Here's how the part is built. I have some questions about the finished solid (model axes, mm). Face numbers are marked on the shaded views. A direction names the side the tool comes from. Give positions to 0.01 mm unless a question says otherwise; leave off trailing zeros. Write each loop counter-clockwise with the first axis right and the second up, starting at its lowest first coordinate (ties: lowest second). Pieces come first, ordered by that corner, then holes. Notation, with made-up numbers: (-31, 66.25) -> (10, 66.25) arc R25 ccw to (10, 97.25) -> close; hole circle Ø4 at (69.5, 8). An arc over 180 degrees is marked (long way). Return JSON: item names as keys, results as strings.
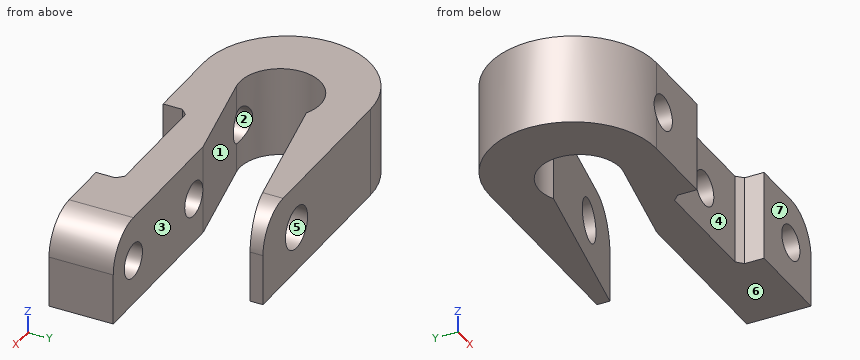
from build123d import *

# Parameters (mm, degrees)
BOSS_EXTRUDE1_DEPTH = 7
CUT_EXTRUDE1_REACH  = 28.495
SKETCH2_R           = 1.35
CUT_EXTRUDE2_REACH  = 28.495
SKETCH3_R           = 1.65
FILLET1_R           = 3
CHAMFER2_SIZE       = 0.5


with BuildPart() as part:
    # Sketch1 → Boss-Extrude1 (new body)
    with BuildSketch(Plane.XY):
        with BuildLine():
            Line((1.443086969, 2.8), (15, 5.5))
            Line((15, 5.5), (15, 6.5))
            Line((15, 6.5), (-1, 6.5))
            ThreePointArc((-1, 6.5), (-7.5, 0), (-1, -6.5))
            Line((-1, -6.5), (5, -6.5))
            Line((5, -6.5), (5, -4.5))
            Line((5, -4.5), (15, -4.5))
            Line((15, -4.5), (15, -6.5))
            Line((15, -6.5), (22, -6.5))
            Line((22, -6.5), (22, -1.5))
            Line((22, -1.5), (8.595407496, -1.5))
            Line((8.595407496, -1.5), (0.615271538, -3.089326939))
            ThreePointArc((0.615271538, -3.089326939), (-3.119335327, 0.438459937), (1.443086969, 2.8))
        make_face()
    extrude(amount=BOSS_EXTRUDE1_DEPTH)

    # Sketch2 → Cut-Extrude1 (cut, up to next)
    with BuildSketch(Plane.XZ.offset(6.5), mode=Mode.PRIVATE) as cut_extrude1_sk1:
        with Locations(Location((0, 3.5, 0), (0, 0, 62.886368109))):
            Circle(SKETCH2_R)
    cut_extrude1_tool1 = extrude(cut_extrude1_sk1.sketch, amount=-CUT_EXTRUDE1_REACH, mode=Mode.PRIVATE) & part.part
    # Sketch2 → Cut-Extrude1 (cut, up to next)
    with BuildSketch(Plane.XZ.offset(6.5), mode=Mode.PRIVATE) as cut_extrude1_sk2:
        with Locations((10, 3.5)):
            Circle(SKETCH2_R)
    cut_extrude1_tool2 = extrude(cut_extrude1_sk2.sketch, amount=-CUT_EXTRUDE1_REACH, mode=Mode.PRIVATE) & part.part
    # Sketch2 → Cut-Extrude1 (cut, up to next)
    with BuildSketch(Plane.XZ.offset(6.5), mode=Mode.PRIVATE) as cut_extrude1_sk3:
        with Locations((19, 3.5)):
            Circle(SKETCH2_R)
    cut_extrude1_tool3 = extrude(cut_extrude1_sk3.sketch, amount=-CUT_EXTRUDE1_REACH, mode=Mode.PRIVATE) & part.part
    add(cut_extrude1_tool1.solids().sort_by_distance((0, -6.5, 3.5))[0], mode=Mode.SUBTRACT)
    add(cut_extrude1_tool2.solids().sort_by_distance((10, -6.5, 3.5))[0], mode=Mode.SUBTRACT)
    add(cut_extrude1_tool3.solids().sort_by_distance((19, -6.5, 3.5))[0], mode=Mode.SUBTRACT)

    # Cut-Extrude2: up to this plane
    cut_extrude2_end = Plane(origin=(1.443086969, 2.8, 7), z_dir=(-0.19532429785675304, 0.9807387107006466, 0))
    # Sketch3 → Cut-Extrude2 (cut, up to the surface)
    with BuildSketch(Plane(origin=(0, 6.5, 0), x_dir=(1, 0, 0), z_dir=(0, 1, 0)), mode=Mode.PRIVATE) as cut_extrude2_sk1:
        with Locations(Location((10, -3.5, 0), (0, 0, 180))):
            Circle(SKETCH3_R)
    cut_extrude2_tool1 = split(extrude(cut_extrude2_sk1.sketch, amount=-CUT_EXTRUDE2_REACH, mode=Mode.PRIVATE), bisect_by=cut_extrude2_end, keep=Keep.BOTH, mode=Mode.PRIVATE)
    add(cut_extrude2_tool1.solids().sort_by_distance((10, 6.5, 3.5))[0], mode=Mode.SUBTRACT)

    # Fillet1
    fillet1_edges = [part.edges().sort_by_distance(p)[0] for p in [
        (15, 6, 7),
        (22, -4, 7),
    ]]
    fillet(fillet1_edges, radius=FILLET1_R)

    # Chamfer2
    chamfer2_edges = [part.edges().sort_by_distance(p)[0] for p in [
        (15, -4.5, 3.5),
        (5, -4.5, 3.5),
    ]]
    chamfer(chamfer2_edges, length=CHAMFER2_SIZE)


solid = part.part
1. Which directions (+Z, -Z, +X, -X, +Y, -Y) give clear straight access to the entire face, cutting with the end or side of a thin tool? Please do the marked faces 1, 2, 3 and 4.
Taken from the geometry:
{"face 1": "+Z, -Z", "face 2": "-Y", "face 3": "+Z, -Z, +X", "face 4": "+Z, -Z, -Y"}
2. For pin 1 Ø1 at (y, z) = (1, 5) entering from -X; pin 2 Ø1.1 at (y, z) = (6, 2) entering from +X; pin 3 Ø1.2 at (y, z) = (-6, 2.5) entering from -X, each with a flat end and sliding along its axis, tell me the tip position at first contact or that it passes through.
Taken from the geometry:
{"pin 1": "stops at x = -7.48", "pin 2": "stops at x = 15", "pin 3": "stops at x = -4.62"}
3. If I drill on line 1 (X direction, y = -3, z = 3); line 2 (Z direction, x = 10, y = 5.45); line 3 (Z direction, x = 10, y = -3.5), over which ranges is the centre line in solid material (lowest first)? Write a range as [from, to].
Taken from the geometry:
{"line 1": "x = [-6.77, -1.25], [1.25, 8.75], [11.25, 17.75], [20.25, 22]", "line 2": "z = [0, 1.85], [5.15, 7]", "line 3": "z = [0, 2.15], [4.85, 7]"}
4. Suppose I cut it at C-C, the plane x = 10. List the corners of the cut face in (y, z) for me.
Taken from the geometry:
{"outline": "(-4.5, 0) -> (-1.5, 0) -> (-1.5, 2.15) -> (-4.5, 2.15) -> close; (-4.5, 4.85) -> (-1.5, 4.85) -> (-1.5, 7) -> (-4.5, 7) -> close; (4.5, 0) -> (6.5, 0) -> (6.5, 1.85) -> (4.5, 1.85) -> close; (4.5, 5.15) -> (6.5, 5.15) -> (6.5, 7) -> (4.5, 7) -> close"}
5. Suppose I cut it at D-D, the plane y = 0. List the corners of the cut face in (x, z) for me, and give its area (4 significant figures).
Taken from the geometry:
{"outline": "(-7.5, 0) -> (-3.15, 0) -> (-3.15, 7) -> (-7.5, 7) -> close", "area": "30.45 mm²"}
6. If we mould it in two halves opening along Z, with no side actions, what happens to the marked faces 5, 6 and 7? For each: released by +Z, released by -Z, zero draft, split by the parting line, or undercut.
Taken from the geometry:
{"face 5": "undercut", "face 6": "released by -Z", "face 7": "zero draft"}
7. Suppose I cut it at A-A, the plane x = 0. List the corners of the cut face in (y, z) for me, and give its area (3 significant figures).
Taken from the geometry:
{"outline": "(-6.5, 0) -> (-3.15, 0) -> (-3.15, 2.15) -> (-6.5, 2.15) -> close; (-6.5, 4.85) -> (-3.15, 4.85) -> (-3.15, 7) -> (-6.5, 7) -> close; (3.15, 0) -> (6.5, 0) -> (6.5, 7) -> (3.15, 7) -> close", "area": "37.9 mm²"}
8. Suppose I cut it at B-B, the plane z = 3. Count the separate pieces of the cut face and the enclosed holes in it, and give its area (3 significant figures).
Taken from the geometry:
{"separate pieces": "5", "enclosed holes": "0", "area": "149 mm²"}
